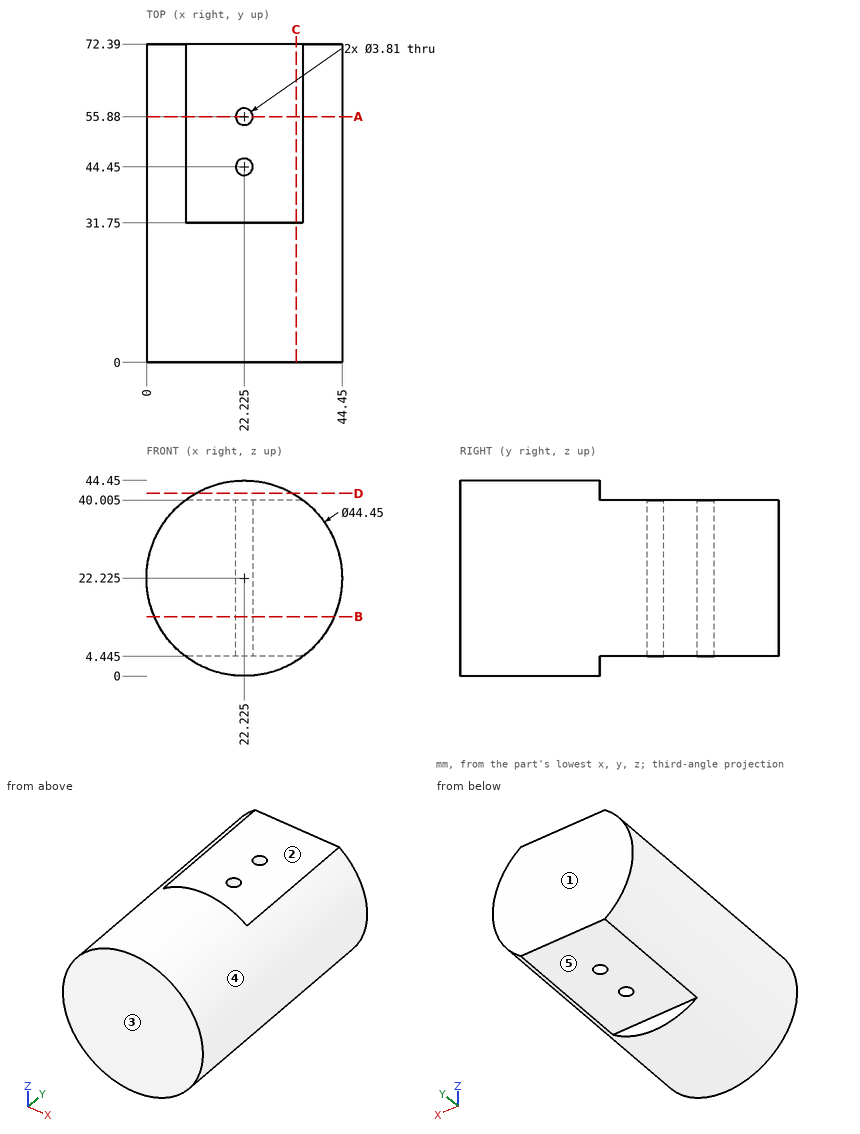
The figure shows three views and two pictorial views of one solid part (mm, origin at its lowest corner). Answer the questions. A direction names the side the tool comes from. Give positions to 0.01 mm unless a question says otherwise; leave off trailing zeros. Loops run counter-clockwise (first coordinate to the right, second up) from the corner with the lowest first, then second, coordinate; pieces in that order, holes last. Notation, with made-up numbers: (-40, 75.5) - (-27, 75.5) arc R28 ccw to (-27, 102.5) - close; hole circle Ø3 at (-22.5, 62). An arc over 180 degrees is marked (long way). Answer in a Markdown table with one row per item.
(1) Consider L1, parallel to Y at x = 29, z = 3; L2, parallel to Z at x = 15, y = 37.5 (3 decimals); L3, parallel to X at y = 23.5, z = 20.5. Determine where each line is inside the solid, lowest interval first. Write a range as [from, to].
Results list:
| item | result |
|---|---|
| L1 | y = [0, 31.75] |
| L2 | z = [4.445, 40.005] |
| L3 | x = [0.07, 44.38] |
(2) Flat-ended cylindrical pins translate along their axes: pin 1 Ø1 at (x, y) = (14.5, 18) entering from -Z; pin 2 Ø6 at (y, z) = (59, 27.5) entering from +X; pin 3 Ø2 at (x, y) = (18.5, 18.5) entering from -Z. Find the tip coordinate at first contact, or state that the pin passes through.
Results list:
| item | result |
|---|---|
| pin 1 | stops at z = 1.21 |
| pin 2 | stops at x = 44.33 |
| pin 3 | stops at z = 0.17 |
(3) Section D-D (z = 41.5) is taken. Give the vertices of the cut face in (x, y), and give its area (3 significant figures).
Results list:
| item | result |
|---|---|
| outline | (11.16, 0) - (33.29, 0) - (33.29, 31.75) - (11.16, 31.75) - close |
| area | 703 mm² |
(4) Section A-A (y = 55.88) is taken. Give the vertices of the cut face in (x, z) (3 decimals).
Results list:
| item | result |
|---|---|
| outline | (8.89, 4.445) - (20.32, 4.445) - (20.32, 40.005) - (8.89, 40.005) arc R22.225 ccw to start; (24.13, 4.445) - (35.56, 4.445) arc R22.225 ccw to (35.56, 40.005) - (24.13, 40.005) - close |
(5) For a pull along Y with two mould halves and no side action, classify the marked faces 1, 2 and 3 as pulls with the +Y half, pulls with the -Y half, needs draft (parallel to the pull), parting line crosses it, or undercut.
Results list:
| item | result |
|---|---|
| face 1 | pulls with the +Y half |
| face 2 | needs draft |
| face 3 | pulls with the -Y half |
(6) Section C-C (x = 34) is taken. Give the vertices of the cut face in (y, z) (3 decimals).
Results list:
| item | result |
|---|---|
| outline | (0, 3.376) - (31.75, 3.376) - (31.75, 4.445) - (72.39, 4.445) - (72.39, 40.005) - (31.75, 40.005) - (31.75, 41.074) - (0, 41.074) - close |
(7) A tool of negligible diameter and unlimited length cuts with its end or side. For the marked faces 4 and 5, from which of +Z, -Z, +X, -X, +Y, -Y can it reach the whole face along a straight path? Write none if from no direction.
Results list:
| item | result |
|---|---|
| face 4 | +Y, -Y |
| face 5 | -Z, +X, -X, +Y |
(8) Section B-B (z = 13.5) is taken. Give the vertices of the cut face in (x, y) (3 decimals).
Results list:
| item | result |
|---|---|
| outline | (1.784, 0) - (42.666, 0) - (42.666, 72.39) - (1.784, 72.39) - close; hole circle Ø3.81 at (22.225, 44.45); hole circle Ø3.81 at (22.225, 55.88) |
